Answer from the drawing. Dimensions are ordinates in mm from the lowest x, y and z of the part. Coordinates: 2 decimals unless noted, no trailing zeros. Write each loop counter-clockwise with the first axis right and the second up, starting at its lowest first coordinate (ties: lowest second). Pieces come first, ordered by that corner, then holes.
1) The part is cut by section D-D (y = 77.5). Determine the outline of the cut face in (x, z).
2) This flat-tipped pin is pushed along its axis until it touches: pin 1 Ø3 at (x, y) = (3, 50) entering from -Z. Where does it stop, or does it pass through?
3) The part is cut by section C-C (y = 44.5). Determine the outline of the cut face in (x, z).
4) The part is cut by section B-B (z = 5.75). Determine the outline of the cut face in (x, y), then the cut area to 3 significant figures.
5) The part is cut by section A-A (x = 8). Determine the outline of the cut face in (y, z).
6) Determine the mould class of the marked faces 1, 2 and 3 for opening direction Y: +Y half, -Y half, draft (parallel to the pull), parting line (faces both ways), or undercut.
7) Find the intervals of material crossed by line 1 (Y direction, x = 10.75, z = 2.5); line 2 (X direction, y = 35.5, z = 7.5); line 3 (X direction, y = 19, z = 11), in increasing order.
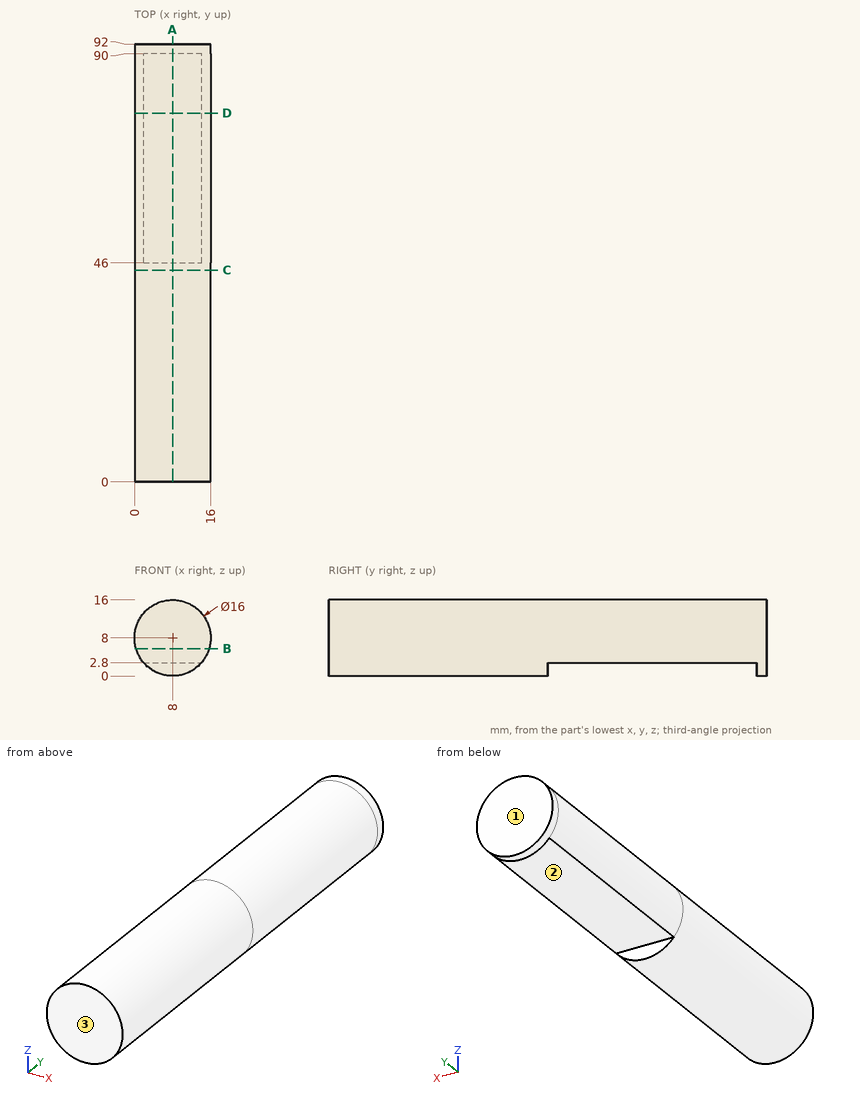
Reported:
1. outline: (1.92, 2.8) - (14.08, 2.8) arc R8 ccw (long way) to start
2. pin 1: stops at z = 2.8
3. outline: circle Ø16 at (8, 8)
4. outline: (0.32, 0) - (15.68, 0) - (15.68, 92) - (0.32, 92) - close
4. area: 1,410 mm2
5. outline: (0, 0) - (46, 0) - (46, 2.8) - (90, 2.8) - (90, 0) - (92, 0) - (92, 16) - (0, 16) - close
6. face 1: +Y half
6. face 2: undercut
6. face 3: -Y half
7. line 1: y = 0 to 46, 90 to 92
7. line 2: x = 0.02 to 15.98
7. line 3: x = 0.58 to 15.42
